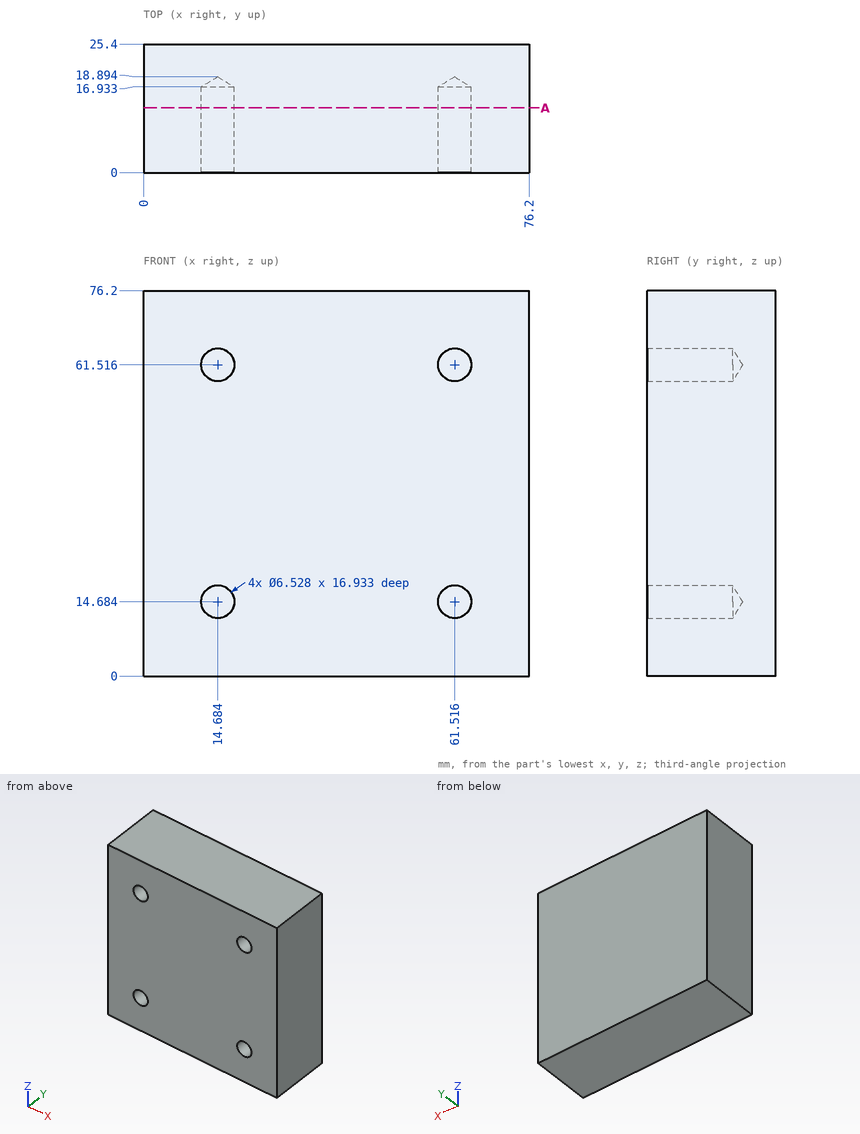
Geometry check sheet. Reference: drawing and pictorial views, mm from the part's lowest x, y, z. Give positions to 0.01 mm unless a question says otherwise; leave off trailing zeros. Write each loop counter-clockwise with the first axis right and the second up, starting at its lowest first coordinate (ties: lowest second). Pieces come first, ordered by that corner, then holes. Notation, with made-up numbers: (27, -29) -> (77, -29) arc R15 cw to (77, -22) -> close; hole circle Ø3 at (39, 84.5). An arc over 180 degrees is marked (long way). One line per question, with ' | ' between items.
Item 1: Scan lines: line 1 along X through (y, z) = (4, 15.5) (1 decimal); line 2 along Z through (x, y) = (59, 14) (1 decimal); line 3 along Z through (x, y) = (62, 5). Record each from-to range of solid material in increasing order.
Determined:
line 1: 0 to 11.5, 17.8 to 58.4, 64.7 to 76.2 | line 2: 0 to 12.6, 16.8 to 59.4, 63.6 to 76.2 | line 3: 0 to 11.46, 17.91 to 58.29, 64.74 to 76.2
Item 2: Sectioned sample at A-A, the plane y = 12.75. Record the boundary of the cut face in (x, z) (1 decimal).
Determined:
outline: (0, 0) -> (76.2, 0) -> (76.2, 76.2) -> (0, 76.2) -> close; hole circle Ø6.5 at (14.7, 14.7); hole circle Ø6.5 at (14.7, 61.5); hole circle Ø6.5 at (61.5, 14.7); hole circle Ø6.5 at (61.5, 61.5)
Item 3: Depth check by flat-ended pin: pin 1 (4 mm diameter, centred on x = 61.52, z = 14.68, fed in from -Y); pin 2 (1.5 mm diameter, centred on x = 19, y = 18, fed in from -Z); pin 3 (5 mm diameter, centred on x = 61.52, z = 61.52, fed in from -Y). Enter the tip coordinate at first touch or a pass-through.
Determined:
pin 1: y = 17.69 | pin 2: z = 0 | pin 3: y = 17.39
